Solid Edge part; units mm, degrees
sketch "Sketch1" plane through (0, 0, 0) normal (0, -1, 0) x (1, 0, 0)
  circle A0 centre (-33.5391, 14.6196) radius 9.375
extrude "Protrusion1" add sketch "Sketch1" against normal blind 40
sketch "Sketch2" plane through (-33.5391, 0, 14.6196) normal (0, -1, 0) x (1, 0, 0)
  circle A0 centre (0, 0) radius 9
extrude "ExtrudedProtrusion_2" add sketch "Sketch2" along normal blind 10 and the other way blind 50.5
fillet "Round_1" radius 1.5 2 edges at (-42.5391, -10, 14.6196) (-42.5391, 50.5, 14.6196)
sketch "Sketch3" plane through (-33.5391, 40, 14.6196) normal (0, 1, 0) x (1, 0, 0)
  line L0 (-6, -11.6345) -> (-6, -6.7082)
  arc A0 (-6, -6.7082) -> (-6, 6.7082) centre (0, 0) cw
  line L1 (-6, 6.7082) -> (-6, 9.3463)
  line L2 (-7, 9.3463) -> (-6, 9.3463)
  line L3 (-7, 7.1414) -> (-7, 9.3463)
  arc A1 (-7, -7.1414) -> (-7, 7.1414) centre (0, 0) cw
  line L4 (-7, -12.6345) -> (-7, -7.1414)
  line L5 (7, -12.6345) -> (-7, -12.6345)
  line L6 (7, -7.1414) -> (7, -12.6345)
  arc A2 (7, 7.1414) -> (7, -7.1414) centre (0, 0) cw
  line L7 (7, 9.3463) -> (7, 7.1414)
  line L8 (6, 9.3463) -> (7, 9.3463)
  line L9 (6, 6.7082) -> (6, 9.3463)
  line L10 (6, -11.6345) -> (6, -6.7082)
  line L11 (-6, -11.6345) -> (6, -11.6345)
  arc A3 (6, 6.7082) -> (6, -6.7082) centre (0, 0) cw
extrude "ExtrudedProtrusion_3" add sketch "Sketch3" along normal blind 7.1438
sketch "Sketch4" plane through (-33.5391, 47.1437, 16.2637) normal (0, 1, 0) x (1, 0, 0)
  line L0 (7, -9.9904) -> (-7, -9.9904)
  line L1 (-7, -9.9904) -> (-7, -10.9904)
  line L2 (-7, -10.9904) -> (7, -10.9904)
  line L3 (7, -10.9904) -> (7, -9.9904)
extrude "ExtrudedProtrusion_4" add sketch "Sketch4" along normal blind 12.5
fillet "Round_2" radius 1.5 6 edges at (-40.0391, 47.1437, 5.2733) (-40.0391, 40, 5.2733) (-27.0391, 40, 5.2733) (-27.0391, 47.1437, 5.2733) (-26.5391, 59.6437, 26.7541) (-40.5391, 59.6437, 26.7541)
mirror "Mirror1" about plane through (0, 20, 0) normal (0, -1, 0) of "ExtrudedProtrusion_4", "ExtrudedProtrusion_3"
fillet "Round1" radius 1.5 6 edges at (-40.0391, -7.1438, 5.2733) (-40.0391, 0, 5.2733) (-27.0391, 0, 5.2733) (-27.0391, -7.1438, 5.2733) (-26.5391, -19.6437, 26.7541) (-40.5391, -19.6437, 26.7541)
sketch "Sketch5" plane through (-33.5391, 49.8219, 27.2541) normal (0, 0, 1) x (1, 0, 0)
  line L0 (12, 13.1801) -> (12, -72.823)
  line L1 (12, -72.823) -> (-12, -72.823)
  line L2 (-12, 13.1801) -> (-12, -72.823)
  line L3 (-12, 13.1801) -> (12, 13.1801)
  dimension "D1" = 12
extrude "ExtrudedProtrusion_7" add sketch "Sketch5" along normal blind 5
chamfer "Chamfer_1" distance 2 angle 45 4 edges at (-33.5391, 63.002, 27.2541) (-45.5391, 20.0004, 27.2541) (-33.5391, -23.0011, 27.2541) (-21.5391, 20.0004, 27.2541)
sketch "Sketch6" plane through (-33.5391, 49.8219, 26.2541) normal (0, 0, -1) x (0, -1, 0)
  line L0 (62.6717, 2.5) -> (62.6717, -2.5)
  line L1 (62.6717, -2.5) -> (67.6717, -2.5)
  line L2 (67.6717, -2.5) -> (67.6717, 2.5)
  line L3 (67.6717, 2.5) -> (62.6717, 2.5)
  line L4 (-8.0189, 2.5) -> (-8.0189, -2.5)
  line L5 (-8.0189, -2.5) -> (-3.0189, -2.5)
  line L6 (-3.0189, -2.5) -> (-3.0189, 2.5)
  line L7 (-3.0189, 2.5) -> (-8.0189, 2.5)
extrude "ExtrudedProtrusion_8" add sketch "Sketch6" along normal blind 6
sketch "Sketch7" plane through (0, 59.6437, 0) normal (0, -1, 0) x (1, 0, 0)
  circle A0 centre (-33.5391, 23.6196) radius 1.5
extrude "Cutout1" cut sketch "Sketch7" along normal up to next
sketch "Sketch8" plane through (-33.5391, 55.3408, 20.2541) normal (0, 0, -1) x (1, 0, 0)
  circle A0 centre (0, 0) radius 1.5
extrude "ExtrudedProtrusion_9" add sketch "Sketch8" along normal blind 1.5
sketch "Sketch9" plane through (-33.5391, -17.8499, 23.2541) normal (0, -1, 0) x (-1, 0, 0)
  circle A0 centre (0, -0.3655) radius 1.5
extrude "Cutout2" cut sketch "Sketch9" against normal up to next
sketch "Sketch10" plane through (-33.5391, -15.3499, 20.2541) normal (0, 0, -1) x (0, -1, 0)
  circle A0 centre (0, 0) radius 1.5
extrude "ExtrudedProtrusion_10" add sketch "Sketch10" along normal blind 1.5
The listing builds one solid part. Answer for the finished solid, in the listing's coordinates (mm). A direction names the side the tool comes from. Coordinates: 2 decimals unless noted, no trailing zeros. Order: outer loops, then holes, each group sorted by start corner. A loop starts at its lowest first (then second) coordinate and runs counter-clockwise, first axis right, second up. Notation, with made-up numbers: M 4,58 L 52,58 A8 ccw 52,67 Z; hole C -37.75,76 d9. An arc over 180 degrees is marked long. Answer as a JSON object with one key per item and string values. Group by question number.
1. Determine the mould class of faces 4 (the flat face through (-34, -15, 18.754)), 5 (the flat face through (-32, 52.841, 23)), 6 (the flat face through (-24, -7.144, 16)) for opening direction Y: released by +Y, released by -Y, zero draft, split by the parting line, or undercut.
2. A tool of negligible diameter and unlimited length cuts with its end or side. For faces 1 (the cylindrical face through (-29.386, -4.19, 22.604)), 2 (the cylindrical face through (-40.03, 40.43, 5.72)), 3 (the flat face through (-31.039, -15, 23)), from which of +Z, -Z, +X, -X, +Y, -Y can it reach the whole face along a straight path? Write none if from no direction.
3. Straight lines are drawn through the part: line 1 (Z direction, x = -27, y = 4); line 2 (Y direction, x = -42.75, z = 17.75); line 3 (Y direction, x = -29.5, z = 19). For each, find the intervals that lie inside material, in ascending order.
4. Flat-ended cylindrical pins translate along their axes: P1, Ø3, axis at x = -25.5, z = 14, coming from the -Y side; P2, Ø3.5, axis at x = -33.5, y = -14.5, coming from the -Z side; P3, Ø0.8, axis at x = -31, z = 23.5, coming from the +Y side; P4, Ø8, axis at x = -34, y = 12.5, coming from the -Z side. Find the tip coordinate at first contact, or state that the pin passes through.
5. Section B-B on y = 24.5 is taken. Write down the section's boundary in (x, z) (3 decimals).
6. Section A-A on y = 48 is taken. Write down the section's boundary in (x, z).
Values follow:
{
 "1": {"face 4": "zero draft", "face 5": "undercut", "face 6": "released by -Y"},
 "2": {"face 1": "none", "face 2": "-Z, -X", "face 3": "-Z, +X, -Y"},
 "3": {"line 1": "7.9 to 21.34, 27.25 to 32.25", "line 2": "-7.14 to 0, 40 to 47.14", "line 3": "-10 to 50.5"},
 "4": {"P1": "y = -10", "P2": "z = 18.75", "P3": "y = 57.84", "P4": "z = 5.24"},
 "5": {"outline": "M -45.539,29.254 L -43.539,27.254 L -23.539,27.254 L -21.539,29.254 L -21.539,32.254 L -45.539,32.254 Z; C -33.539,14.62 d18.75"},
 "6": {"outline": "M -45.54,29.25 L -43.54,27.25 L -40.54,27.25 L -40.54,26.25 L -26.54,26.25 L -26.54,27.25 L -23.54,27.25 L -21.54,29.25 L -21.54,32.25 L -45.54,32.25 Z; C -33.54,14.62 d18"}
}
